Check sheet for the modelled part. Datum: model origin and axes. Units: mm. A direction names the side the tool comes from. Round coordinates to 2 decimals unless told otherwise and drop trailing zeros. Order: outer loops, then holes, each group sorted by start corner. A loop starts at its lowest first (then second) coordinate and runs counter-clockwise, first axis right, second up.
Q1. Mould release check, pull along X, two halves, no side actions. Record for faces 1 (the flat face through (-1, -3, -6)), 2 (the flat face through (2.24, -1.32, -4.52)), 3 (the cylindrical face through (2.5, -0.1, 8.6)): +X half, -X half, draft (parallel to the pull), parting line (faces both ways), or undercut.
Q2. Cross-section at C-C on z = 10.5. Record the cut outline in (x, y), then the cut area to 3 significant figures.
Q3. Cross-section at B-B on x = 0. Record the cut outline in (y, z).
Q4. Depth check by flat-ended pin: P1, Ø1, axis at y = -2.5, z = -3, coming from the +X side; P2, Ø1, axis at x = -3.5, y = 1, coming from the +Z side; P3, Ø3, axis at y = 1, z = 8, coming from the -X side. Enter the tip coordinate at first touch or a pass-through.
Q5. Scan lines: probe 1 along Y at (x, z) = (-2, 9.5); probe 2 along Z at (x, y) = (4, 0.25). Record each from-to range of solid material in increasing order.
Q6. Cross-section at A-A on z = -4.5. Record the cut outline in (x, y).
Q7. Set-up check for faces 4 (the flat face through (-2, -2, 0)), 5 (the flat face through (0, 0, -3)), 6 (the cylindrical face through (1.08, -4.88, -2.71)): record each of +Z, -Z, +X, -X, +Y, -Y from which the full face is reachable in a straight line by a thin tool's end or side.
from build123d import *

# Parameters (mm, degrees)
ESQUISSE1_R             = 2.5
BASE_EXTRUSION_DEPTH    = 18
CHANFREIN1_SIZE         = 0.5
ESQUISSE2_R             = 5
BOSS_EXTRU_1_DEPTH      = 6
ENL_V_MAT_EXTRU_1_DEPTH = 3
ESQUISSE4_R             = 3
ENL_V_MAT_EXTRU_2_DEPTH = 0.5
ENL_V_MAT_EXTRU_2_DRAFT = -45
CONG_1_R                = 0.5


with BuildPart() as part:
    # Esquisse1 → Base-Extrusion (new body)
    with BuildSketch(Plane.XY):
        with Locations(Location((0, 0, 0), (0, 0, 180))):  # turned: the seam where the file's is
            Circle(ESQUISSE1_R)
    extrude(amount=BASE_EXTRUSION_DEPTH)

    # Chanfrein1
    chanfrein1_edges = [part.edges().sort_by_distance(p)[0] for p in [
        (2.5, 0, 18),
    ]]
    chamfer(chanfrein1_edges, length=CHANFREIN1_SIZE)

    # Esquisse2 → Boss.-Extru.1 (add)
    with BuildSketch(Plane(origin=(0, 0, 0), x_dir=(-1, 0, 0), z_dir=(0, 0, -1))):
        Circle(ESQUISSE2_R)
    extrude(amount=BOSS_EXTRU_1_DEPTH)

    # Esquisse3 → Enlèv. mat.-Extru.1 (cut)
    with BuildSketch(Plane(origin=(0, 0, -6), x_dir=(-1, 0, 0), z_dir=(0, 0, -1))):
        Polygon((-3, 0), (-1.5, 2.598076211), (1.5, 2.598076211), (3, 0), (1.5, -2.598076211), (-1.5, -2.598076211), align=None)
    extrude(amount=-ENL_V_MAT_EXTRU_1_DEPTH, mode=Mode.SUBTRACT)


with BuildPart() as enl_v_mat_extru_2_tool:
    # Esquisse4 → Enlèv. mat.-Extru.2 (with draft: the straight prism first)
    with BuildSketch(Plane(origin=(0, 0, -6), x_dir=(-1, 0, 0), z_dir=(0, 0, -1))):
        Circle(ESQUISSE4_R)
    extrude(amount=-ENL_V_MAT_EXTRU_2_DEPTH)
    # Enlèv. mat.-Extru.2: the draft: its side faces are tilted about the plane it starts from
    enl_v_mat_extru_2_sides = [enl_v_mat_extru_2_tool.faces().sort_by_distance(p)[0] for p in [
        (3, 0, -5.75),
    ]]
    draft(enl_v_mat_extru_2_sides, Plane(origin=(0, 0, -6), x_dir=(-1, 0, 0), z_dir=(0, 0, -1)), ENL_V_MAT_EXTRU_2_DRAFT)


with BuildPart() as part_1:
    add(part.part)

    # Enlèv. mat.-Extru.2: cut by enl_v_mat_extru_2_tool
    add(enl_v_mat_extru_2_tool.part, mode=Mode.SUBTRACT)

    # Congé1
    cong_1_edges = [part_1.edges().sort_by_distance(p)[0] for p in [
        (5, 0, -6),
    ]]
    fillet(cong_1_edges, radius=CONG_1_R)


solid = part_1.part
Results found:
1. face 1: draft
1. face 2: undercut
1. face 3: parting line
2. outline: circle Ø5 at (0, 0)
2. area: 19.6 mm2
3. outline: (-5, -5.5) arc R0.5 ccw to (-4.5, -6) - (-3, -6) - (-2.6, -5.6) - (-2.6, -3) - (2.6, -3) - (2.6, -5.6) - (3, -6) - (4.5, -6) arc R0.5 ccw to (5, -5.5) - (5, 0) - (2.5, 0) - (2.5, 17.5) - (2, 18) - (-2, 18) - (-2.5, 17.5) - (-2.5, 0) - (-5, 0) - close
4. P1: stops at x = 4.58
4. P2: stops at z = 0
4. P3: stops at x = -2.5
5. probe 1: y = -1.5 to 1.5
5. probe 2: z = -6 to 0
6. outline: circle Ø10 at (0, 0); hole (-3, 0) - (-1.5, -2.6) - (1.5, -2.6) - (3, 0) - (1.5, 2.6) - (-1.5, 2.6) - close
7. face 4: +Z
7. face 5: -Z
7. face 6: +Z, -Z
